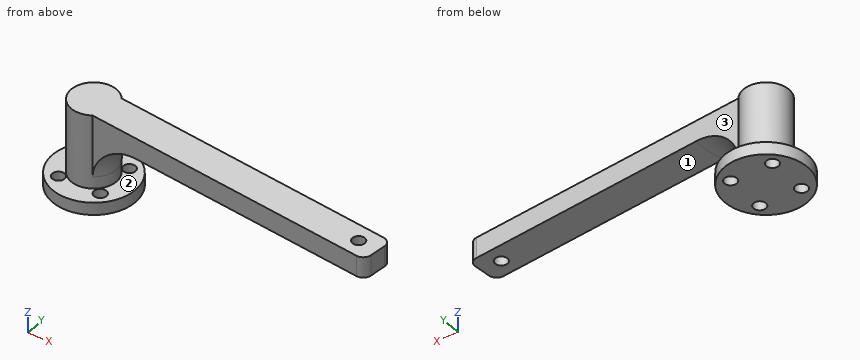
```python
from build123d import *

# Parameters (mm, degrees)
SKETCH_1_R          = 10
EXTRUDE_1_DEPTH     = 3
SKETCH_2_R          = 1.5
CUT_EXTRUDE_1_DEPTH = 15.45683229480096
EXTRUDE_START       = 12.9
SKETCH_3_R          = 5.465897693502911
SKETCH_3_R_2        = 1.5000000000000002
EXTRUDE_2_DEPTH     = 12.9
EXTRUDE_START_2     = -15.9
SKETCH_4_R          = 1.5000000000000002
EXTRUDE_4_DEPTH     = 15.9
EXTRUDE_5_DEPTH     = 5
SKETCH_6_R          = 1.4999999999999973
CUT_EXTRUDE_2_DEPTH = 79.62526207388743
EXTRUDE_START_3     = 5
EXTRUDE_8_DEPTH     = 5
FILLET_1_R          = 10
FILLET_2_R          = 2


with BuildPart() as part:
    # 草图1 → 凸台-拉伸1 (new body)
    with BuildSketch(Plane.XY):
        Circle(SKETCH_1_R)
    extrude(amount=EXTRUDE_1_DEPTH)

    # 草图2 → 切除-拉伸1 (cut, through all)
    with BuildSketch(Plane.XY.offset(3)):
        with BuildLine():
            ThreePointArc((-3.5, 4.999999999999998), (-6.060660171779828, 6.060660171779813), (-4.999999999999981, 3.4999999999999982))
            Line((-5, 3.499999999999999), (-5, 4.999999999999999))
            Line((-5, 4.999999999999998), (-3.5, 4.999999999999998))
        make_face()
        with BuildLine():
            Line((-5, 4.999999999999999), (-5, 3.499999999999999))
            ThreePointArc((-4.999999999999981, 3.4999999999999982), (-3.939339828220172, 3.9393398282201835), (-3.5, 4.999999999999998))
            Line((-3.5, 4.999999999999998), (-5, 4.999999999999998))
        make_face()
        with BuildLine():
            ThreePointArc((3.499999999999999, 5.000000000000001), (3.9393398282201844, 3.939339828220173), (5.000000000000019, 3.5))
            Line((5, 3.500000000000001), (5, 5.000000000000001))
            Line((5, 5.000000000000001), (3.499999999999999, 5.000000000000001))
        make_face()
        with BuildLine():
            Line((5, 5.000000000000001), (5, 3.500000000000001))
            ThreePointArc((5.000000000000019, 3.5), (6.060660171779828, 3.9393398282201852), (6.500000000000001, 5.000000000000001))
            ThreePointArc((6.500000000000001, 5.000000000000001), (5, 6.500000000000002), (3.499999999999999, 5.000000000000001))
            Line((3.499999999999999, 5.000000000000001), (5, 5.000000000000001))
        make_face()
        with BuildLine():
            ThreePointArc((-4.9999999999999805, -3.500000000000001), (-6.060660171779829, -6.060660171779815), (-3.5, -5.000000000000001))
            Line((-3.5, -5.000000000000001), (-5, -5.000000000000001))
            Line((-5, -5.000000000000001), (-5, -3.500000000000001))
        make_face()
        with BuildLine():
            Line((-5, -5.000000000000001), (-3.5, -5.000000000000001))
            ThreePointArc((-3.5, -5.000000000000001), (-3.939339828220172, -3.939339828220186), (-4.9999999999999805, -3.500000000000001))
            Line((-5, -3.500000000000001), (-5, -5.000000000000001))
        make_face()
        with BuildLine():
            ThreePointArc((5.0000000000000195, -3.4999999999999982), (3.9393398282201852, -3.9393398282201706), (3.499999999999999, -4.999999999999999))
            Line((3.499999999999999, -4.999999999999999), (5, -4.999999999999999))
            Line((5, -4.999999999999999), (5, -3.4999999999999982))
        make_face()
        with BuildLine():
            Line((5, -4.999999999999999), (3.499999999999999, -4.999999999999999))
            ThreePointArc((3.499999999999999, -4.999999999999999), (5, -6.5), (6.500000000000001, -4.999999999999999))
            ThreePointArc((6.500000000000001, -4.999999999999999), (6.060660171779829, -3.9393398282201844), (5.0000000000000195, -3.4999999999999982))
            Line((5, -3.4999999999999982), (5, -4.999999999999999))
        make_face()
        Circle(SKETCH_2_R)
    extrude(amount=-CUT_EXTRUDE_1_DEPTH, mode=Mode.SUBTRACT)

    # 草图3 → 凸台-拉伸2 (add)
    with BuildSketch(Plane.XY.offset(3).offset(EXTRUDE_START)):
        with Locations(Location((-0.07436650387235982, 0.07436650387235982, 0), (0, 0, 135))):
            Circle(SKETCH_3_R)
        Circle(SKETCH_3_R_2, mode=Mode.SUBTRACT)
    extrude(amount=-EXTRUDE_2_DEPTH)

    # 草图4 → 凸台-拉伸4 (add)
    with BuildSketch(Plane(origin=(0, 0, 0), x_dir=(-1, 0, 0), z_dir=(0, 0, -1)).offset(EXTRUDE_START_2)):
        Circle(SKETCH_4_R)
    extrude(amount=EXTRUDE_4_DEPTH)

    # 草图5 → 凸台-拉伸5 (add)
    with BuildSketch(Plane.XY.offset(15.9)):
        Polygon((74.67295984530996, -5.059165048643418), (73.72436785298946, -13.002726795876548), (-0.7465235273211024, -4.1096768678718245), (0.2020684649993922, 3.83388487936125), align=None)
    extrude(amount=EXTRUDE_5_DEPTH)

    # 草图6 → 切除-拉伸2 (cut, through all)
    with BuildSketch(Plane.XY.offset(20.900000000000002)):
        with Locations((69.23393775712903, -8.438075927059709)):
            Circle(SKETCH_6_R)
    extrude(amount=-CUT_EXTRUDE_2_DEPTH, mode=Mode.SUBTRACT)

    # 草图7 → 凸台-拉伸8 (add)
    with BuildSketch(Plane.XY.offset(15.9).offset(EXTRUDE_START_3)):
        with BuildLine():
            Line((0.2020684649993922, 3.83388487936125), (4.305897204794468, 3.3438201949921416))
            ThreePointArc((4.305897204794468, 3.3438201949921416), (-5.4500676526118506, 1.0632420042673105), (2.8556757439201084, -4.53983873885273))
            Line((2.8556757439201084, -4.53983873885273), (-0.7465235273211024, -4.1096768678718245))
            Line((-0.7465235273211024, -4.1096768678718245), (0.2020684649993922, 3.83388487936125))
        make_face()
    extrude(amount=-EXTRUDE_8_DEPTH)

    # 圆角1
    fillet_1_edges = [part.edges().sort_by_distance(p)[0] for p in [
        (5.301334644867113, -0.914508996522684, 15.9),
    ]]
    fillet(fillet_1_edges, radius=FILLET_1_R)

    # 圆角2
    fillet_2_edges = [part.edges().sort_by_distance(p)[0] for p in [
        (73.72436785298946, -13.002726795876548, 18.4),
        (74.67295984530996, -5.059165048643418, 18.4),
    ]]
    fillet(fillet_2_edges, radius=FILLET_2_R)


solid = part.part
```
The model under review builds one solid part; all positions refer to its coordinate system, in mm. Face numbers are marked on the shaded views. Round coordinates to 2 decimals unless told otherwise and drop trailing zeros. Write each loop counter-clockwise with the first axis right and the second up, starting at its lowest first coordinate (ties: lowest second). Pieces come first, ordered by that corner, then holes. Notation, with made-up numbers: (-0.75, 7.5) - (17.25, 7.5) arc R21 cw to (17.25, 12.5) - close; hole circle Ø3 at (2, 11). An arc over 180 degrees is marked (long way). Answer as CSV lines item,"result". Start each with the question number.
(1) We need section C-C on x = 40. State the section outline as (y, z) points, plus the area to 3 significant figures.
(2) We need section B-B on z = 7.25. State the section outline as (x, y) points.
(3) We need section A-A on x = 0. State the section outline as (y, z) points, plus the area to 3 significant figures.
(4) To check wall thickness, follow line 1 (Z direction, x = 65, y = -9); line 2 (X direction, y = 5, z = 1); line 3 (Y direction, x = 69, z = 17). State the ranges of each line that lie inside material, in increasing order.
(5) Draft analysis for pull direction Z (two halves, no side actions). For the marked faces 1, 2 and 3, state which applies: pulls with the +Z half, pulls with the -Z half, needs draft (parallel to the pull), parting line crosses it, or undercut.
(6) For pin 1 Ø12 at (x, z) = (-1, 10) entering from +Y; pin 2 Ø3 at (x, z) = (61.5, 17) entering from -Y; pin 3 Ø12 at (x, y) = (31, -9.5) entering from -Z, all flat-tipped, find the tip position at first contact; note any pin that passes through.
Worked answers:
1,outline,"(-8.98, 15.9) - (-0.92, 15.9) - (-0.92, 20.9) - (-8.98, 20.9) - close"
1,area,"40.3 mm²"
2,outline,"(2.86, -4.54) - (3, -4.56) arc R5.56 ccw to (4.43, 3.33) - (4.31, 3.34) arc R5.47 ccw (long way) to start"
3,outline,"(-10, 0) - (10, 0) - (10, 3) - (5.54, 3) - (5.54, 20.9) - (-5.39, 20.9) - (-5.39, 3) - (-10, 3) - close"
3,area,"256 mm²"
4,line 1,"15.9 to 20.9"
4,line 2,"-8.66 to -6.5, -3.5 to 3.5, 6.5 to 8.66"
4,line 3,"-12.44 to -9.92, -6.96 to -4.38"
5,face 1,"pulls with the -Z half"
5,face 2,"undercut"
5,face 3,"needs draft"
6,pin 1,"y = 5.54"
6,pin 2,"y = -11.72"
6,pin 3,"z = 15.9"
